from build123d import *

# Parameters (mm, degrees)
SKETCH1_W           = 86.36
SKETCH1_H           = 8.89
BOSS_EXTRUDE1_DEPTH = 38.1
SKETCH2_R           = 12.7
CUT_EXTRUDE1_DEPTH  = 59.267954315
SKETCH3_R           = 3.175
BOSS_EXTRUDE2_DEPTH = 38.1
SKETCH5_R           = 3.175
CUT_EXTRUDE2_DEPTH  = 1.5875


with BuildPart() as part:
    # Sketch1 → Boss-Extrude1 (new body)
    with BuildSketch(Plane(origin=(0, 0, 0), x_dir=(1, 0, 0), z_dir=(0, 1, 0))):
        Rectangle(SKETCH1_W, SKETCH1_H)
    extrude(amount=BOSS_EXTRUDE1_DEPTH)

    # Sketch2 → Cut-Extrude1 (cut, through all)
    with BuildSketch(Plane.XY.offset(4.445)):
        with Locations((19.05, 19.05)):
            Circle(SKETCH2_R)
        with Locations((-19.05, 19.05)):
            Circle(SKETCH2_R)
    extrude(amount=-CUT_EXTRUDE1_DEPTH, mode=Mode.SUBTRACT)

    # Sketch3 → Boss-Extrude2 (add)
    with BuildSketch(Plane.XZ):
        with Locations(Location((0, 0, 0), (0, 0, 90))):
            Circle(SKETCH3_R)
    extrude(amount=BOSS_EXTRUDE2_DEPTH)

    # Sketch4 → Revolve1 (revolve)
    with BuildSketch(Plane.XZ.offset(38.1)):
        with BuildLine():
            Line((0, -9.525), (0, 9.525))
            ThreePointArc((0, 9.525), (9.525, 0), (0, -9.525))
        make_face()
    revolve(axis=Axis((0, -38.1, -9.525), (0, 0, 1)))

    # Sketch5 → Cut-Extrude2 (cut)
    with BuildSketch(Plane(origin=(43.18, 0, 0), x_dir=(0, 0, -1), z_dir=(1, 0, 0))):
        with Locations((0, 29.21)):
            Circle(SKETCH5_R)
        with Locations(Location((0, 8.89, 0), (0, 0, 180))):
            Circle(SKETCH5_R)
    cut_extrude2 = extrude(amount=-CUT_EXTRUDE2_DEPTH, mode=Mode.SUBTRACT)

    # Mirror1: Cut-Extrude2 across plane
    add(cut_extrude2.mirror(Plane(origin=(0, 0, 0), x_dir=(0, 0, 1), z_dir=(1, 0, 0))), mode=Mode.SUBTRACT)


solid = part.part
Geometry check sheet. Reference: the model listing, model coordinates, mm. A direction names the side the tool comes from. Coordinates: 2 decimals unless noted, no trailing zeros. Order: outer loops, then holes, each group sorted by start corner. A loop starts at its lowest first (then second) coordinate and runs counter-clockwise, first axis right, second up. Notation, with made-up numbers: (-18, 44) - (25, 44) arc R20 ccw to (25, 52) - close; hole circle Ø11 at (37, 77.5). An arc over 180 degrees is marked (long way). Answer in a Markdown table with one row per item. Add a question column.
1) Cross-section at A-A, the plane x = 19.05. Record the cut outline in (y, z) (3 decimals).
2) Cross-section at C-C, the plane z = 0. State how many separate pieces and enclosed holes the cut face has, then the cut area to 3 significant figures.
3) Set-up check for faces 1 (the flat face through (41.592, 29, 0)), 2 (the flat face through (-1, 19, 4.445)), 3 (the cylindrical face through (1.93, -14.36, -2.52)): record each of +Z, -Z, +X, -X, +Y, -Y from which the full face is reachable in a straight line by a thin tool's end or side.
4) Material ranges on line 1 along Y through (x, z) = (-42.65, 0) (3 decimals); line 2 along Y through (x, z) = (19.05, 1.75); line 3 along Z through (x, y) = (42, 29) (3 decimals), recorded low to high. Write a range as [from, to].
5) Cross-section at D-D, the plane y = 8.89. Record the cut outline in (x, z) (1 decimal).
6) Release check for a two-part mould opening along X. For faces 4 (the cylindrical face through (30.782, 14.186, 0.062)), 5 (the flat face through (-41.592, 29, 0)), 6 (the cylindrical face through (-42.397, 26.393, -1.465)) record: +X half, -X half, draft (parallel to the pull), parting line (faces both ways), or undercut.
7) Gauge pin test, flat ends, axial feed: P1, Ø3, axis at x = -10.5, y = 27, coming from the -Z side (3 decimals); P2, Ø6, axis at y = -18, z = 4.5, coming from the +X side; P3, Ø1.9, axis at y = 8, z = -0.5, coming from the +X side. Record the tip position at first contact, or that the pin passes through.
8) Cross-section at B-B, the plane y = 19.05. Record the cut outline in (x, z) (3 decimals).
Check result:
| question | item | result |
|---|---|---|
| 1 | outline | (0, -4.445) - (6.35, -4.445) - (6.35, 4.445) - (0, 4.445) - close; (31.75, -4.445) - (38.1, -4.445) - (38.1, 4.445) - (31.75, 4.445) - close |
| 2 | separate pieces | 1 |
| 2 | enclosed holes | 2 |
| 2 | area | 2,700 mm² |
| 3 | face 1 | +X |
| 3 | face 2 | +Z, +X, -X, +Y |
| 3 | face 3 | none |
| 4 | line 1 | y = [0, 5.715], [12.065, 26.035], [32.385, 38.1] |
| 4 | line 2 | y = [0, 6.35], [31.75, 38.1] |
| 4 | line 3 | z = [-4.445, -3.168], [3.168, 4.445] |
| 5 | outline | (-43.2, -4.4) - (-26.7, -4.4) - (-26.7, 4.4) - (-43.2, 4.4) - (-43.2, 3.2) - (-41.6, 3.2) - (-41.6, -3.2) - (-43.2, -3.2) - close; (-11.4, -4.4) - (11.4, -4.4) - (11.4, 4.4) - (-11.4, 4.4) - close; (26.7, -4.4) - (43.2, -4.4) - (43.2, -3.2) - (41.6, -3.2) - (41.6, 3.2) - (43.2, 3.2) - (43.2, 4.4) - (26.7, 4.4) - close |
| 6 | face 4 | undercut |
| 6 | face 5 | -X half |
| 6 | face 6 | draft |
| 7 | P1 | stops at z = -4.445 |
| 7 | P2 | stops at x = 2.8 |
| 7 | P3 | stops at x = 41.59 |
| 8 | outline | (-43.18, -4.445) - (-31.75, -4.445) - (-31.75, 4.445) - (-43.18, 4.445) - close; (-6.35, -4.445) - (6.35, -4.445) - (6.35, 4.445) - (-6.35, 4.445) - close; (31.75, -4.445) - (43.18, -4.445) - (43.18, 4.445) - (31.75, 4.445) - close |
